from build123d import *

# Parameters (mm, degrees)
EXTRUDE_1_DEPTH     = 400
FILLET_1_R          = 0.8
SKETCH_2_R          = 2
CUT_EXTRUDE_1_DEPTH = 2
SKETCH_3_R          = 2
CUT_EXTRUDE_2_DEPTH = 400


with BuildPart() as part:
    # 草图1 → 凸台-拉伸1 (new body)
    with BuildSketch(Plane.XY):
        Polygon((0, 0), (0, 15), (-2, 15), (-2, 2), (-15, 2), (-15, 0), align=None)
    extrude(amount=EXTRUDE_1_DEPTH)

    # 圆角1
    fillet_1_edges = [part.edges().sort_by_distance(p)[0] for p in [
        (-15, 2, 200),
        (-2, 15, 200),
    ]]
    fillet(fillet_1_edges, radius=FILLET_1_R)

    # 草图2 → 切除-拉伸1 (cut)
    with BuildSketch(Plane(origin=(0, 2, 0), x_dir=(1, 0, 0), z_dir=(0, 1, 0))):
        with Locations((-8, -222)):
            Circle(SKETCH_2_R)
    extrude(amount=-CUT_EXTRUDE_1_DEPTH, mode=Mode.SUBTRACT)

    # 草图3 → 切除-拉伸2 (cut)
    with BuildSketch(Plane.ZY.offset(2)):
        with Locations((390, 9)):
            Circle(SKETCH_3_R)
    extrude(amount=-CUT_EXTRUDE_2_DEPTH, mode=Mode.SUBTRACT)


solid = part.part
For this review, take the finished solid that the model builds, in its own axes (mm). A direction names the side the tool comes from. Coordinates: 2 decimals unless noted, no trailing zeros. Loops run counter-clockwise (first coordinate to the right, second up) from the corner with the lowest first, then second, coordinate; pieces in that order, holes last. Notation, with made-up numbers: (-33, 69.5) - (7, 69.5) arc R14 cw to (7, 87.5) - close; hole circle Ø11 at (1.25, 66.5). An arc over 180 degrees is marked (long way). Use a Markdown table: item, result. Add a question column.
Item 1: Insertion check: pin 1 Ø1 at (y, z) = (11, 92) entering from -X; pin 2 Ø3.5 at (y, z) = (9, 390) entering from +X; pin 3 Ø6.5 at (x, z) = (-8, 222) entering from +Y. Each pin has a flat end and moves straight along its axis. Give the tip position at first contact, or say it passes through.
Item 2: We need section A-A (z = 74.5). Give the boundary of the cut face in (x, y).
Item 3: For line 1 (X direction, y = 0.6, z = 222); line 2 (Y direction, x = -1.45, z = 390); line 3 (X direction, y = 10, z = 140), list the stretches that pass through material, from the lowest coordinate up.
Item 4: Tool access review of faces 1 (the face through (0, 7, 197)), 2 (the face through (-8, 2, 197)): name each direction out of +Z, -Z, +X, -X, +Y, -Y from which nothing blocks a thin tool from reaching the whole face with its end or side.
Results list:
| question | item | result |
|---|---|---|
| 1 | pin 1 | stops at x = -2 |
| 1 | pin 2 | passes through |
| 1 | pin 3 | stops at y = 2 |
| 2 | outline | (-15, 0) - (0, 0) - (0, 15) - (-1.2, 15) arc R0.8 ccw to (-2, 14.2) - (-2, 2) - (-14.2, 2) arc R0.8 ccw to (-15, 1.2) - close |
| 3 | line 1 | x = -15 to -10, -6 to 0 |
| 3 | line 2 | y = 0 to 7, 11 to 14.96 |
| 3 | line 3 | x = -2 to 0 |
| 4 | face 1 | +Z, -Z, +X, +Y, -Y |
| 4 | face 2 | +Z, -Z, -X, +Y |
